```python
from build123d import *

# Parameters (mm, degrees)
CROQUIS2_R              = 25.443991431
CROQUIS2_R_2            = 10
SALIENTE_EXTRUIR1_DEPTH = 20


with BuildPart() as part:
    # Croquis1 → Revolución1 (revolve)
    with BuildSketch(Plane.XY, mode=Mode.PRIVATE) as revoluci_n1_sk:
        Polygon((100, 5), (100, -5), (111.6503736, -12.670841247), (111.6503736, -12.7), (88.202160832, -12.7), (80.211990776, -7.5), (28.828149692, -7.5), (25.443991431, -12.7), (10, -12.7), (10, 12.7), (25.443991431, 12.7), (28.828149692, 7.5), (80.211990776, 7.5), (88.202160832, 12.7), (111.6503736, 12.7), (111.6503736, 12.670841247), align=None)
    revolve(revoluci_n1_sk.sketch.rotate(Axis((0, -23.836508292, 0), (0, 1, 0)), 90), axis=Axis((0, -23.836508292, 0), (0, 1, 0)))

    # Croquis2 → Saliente-Extruir1 (add)
    with BuildSketch(Plane.XZ.offset(12.7)):
        with Locations(Location((0, 0, 0), (0, 0, 270))):
            Circle(CROQUIS2_R)
        with Locations(Location((0, 0, 0), (0, 0, 270))):
            Circle(CROQUIS2_R_2, mode=Mode.SUBTRACT)
    extrude(amount=SALIENTE_EXTRUIR1_DEPTH)


solid = part.part
```
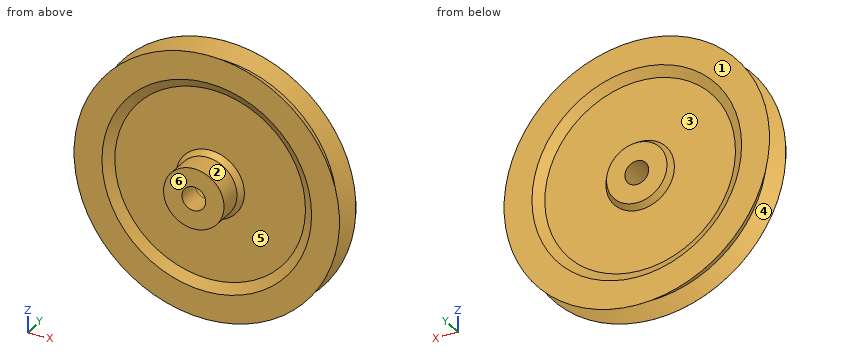
Read the model definition and answer for the solid it produces. Units are mm, in the model's axes. Face numbers are marked on the shaded views. A direction names the side the tool comes from. Give positions to 0.01 mm unless a question says otherwise; leave off trailing zeros. Write each loop counter-clockwise with the first axis right and the second up, starting at its lowest first coordinate (ties: lowest second). Pieces come first, ordered by that corner, then holes. Notation, with made-up numbers: (23.5, -32) -> (82.5, -32) arc R30 ccw to (82.5, 2) -> close; hole circle Ø8 at (-5.75, 78.5). An arc over 180 degrees is marked (long way). Answer as a JSON object with one key per item and string values.
1) For a pull along Z with two mould halves and no side action, classify the marked faces 1, 2 and 3 as pulls with the +Z half, pulls with the -Z half, needs draft (parallel to the pull), parting line crosses it, or undercut.
Findings below:
{"face 1": "needs draft", "face 2": "parting line crosses it", "face 3": "undercut"}
2) Section C-C on y = -22 is taken. Write down the section's boundary in (x, z).
Findings below:
{"outline": "circle Ø50.89 at (0, 0); hole circle Ø20 at (0, 0)"}
3) Flat-ended cylindrical pins translate along their axes: pin 1 Ø10 at (x, z) = (82.5, 26.5) entering from -Y; pin 2 Ø10 at (x, z) = (-47.5, 46.5) entering from +Y; pin 3 Ø10 at (x, y) = (28, 0) entering from +Z. Find the tip coordinate at first contact, or state that the pin passes through.
Findings below:
{"pin 1": "stops at y = -12.7", "pin 2": "stops at y = 7.5", "pin 3": "stops at z = 97.32"}
4) Straight lines are drawn through the part: probe 1 along X at (y, z) = (-28.5, 0); probe 2 along X at (y, z) = (0, 0). For each, find the intervals that lie inside material, in ascending order. Write a range as from..to.
Findings below:
{"probe 1": "x = -25.44..-10, 10..25.44", "probe 2": "x = -100..-10, 10..100"}
5) A tool of negligible diameter and unlimited length cuts with its end or side. For the marked faces 4, 5 and 6, from which of +Z, -Z, +X, -X, +Y, -Y can it reach the whole face along a straight path? Write none if from no direction.
Findings below:
{"face 4": "none", "face 5": "-Y", "face 6": "+Z, -Z, +X, -X, -Y"}
